```python
from build123d import *

# Parameters (mm, degrees)
SKETCH_W        = 24
SKETCH_H        = 5
PAD_DEPTH       = 5
SKETCH001_R     = 3.75
POCKET_DEPTH    = 2
SKETCH002_R     = 3.75
POCKET001_DEPTH = 2
SKETCH003_R     = 4
POCKET002_DEPTH = 5
SKETCH004_R     = 1.51
POCKET003_DEPTH = 3


with BuildPart() as part:
    # Sketch → Pad (new body)
    with BuildSketch(Plane.XY):
        Rectangle(SKETCH_W, SKETCH_H)
    extrude(amount=PAD_DEPTH)

    # Sketch001 (on Face3 of Pad) → Pocket (cut)
    with BuildSketch(Plane.XZ.offset(2.5)):
        with Locations((0, -2)):
            Circle(SKETCH001_R)
    extrude(amount=-POCKET_DEPTH, mode=Mode.SUBTRACT)

    # Sketch002 (on Face1 of Pocket) → Pocket001 (cut)
    with BuildSketch(Plane(origin=(0, 2.5, 0), x_dir=(-1, 0, 0), z_dir=(0, 1, 0))):
        with Locations((0, -2)):
            Circle(SKETCH002_R)
    extrude(amount=-POCKET001_DEPTH, mode=Mode.SUBTRACT)

    # Sketch003 (on Face7 of Pocket001) → Pocket002 (cut)
    with BuildSketch(Plane.XZ.offset(2.5)):
        with Locations((0, -3)):
            Circle(SKETCH003_R)
        with BuildLine():
            ThreePointArc((4.021194, 2.8), (0, 4.9), (-4.021194, 2.8))
            Line((-4.021194, 2.8), (-12, 2.8))
            Line((-12, 2.8), (-12, 5))
            Line((-12, 5), (12, 5))
            Line((12, 2.8), (12, 5))
            Line((4.021194, 2.8), (12, 2.8))
        make_face()
    extrude(amount=-POCKET002_DEPTH, mode=Mode.SUBTRACT)

    # Sketch004 (on Face8 of Pocket002) → Pocket003 (cut)
    with BuildSketch(Plane.XY.offset(2.8)):
        with Locations((-8, 0)):
            Circle(SKETCH004_R)
        with Locations((8, 0)):
            Circle(SKETCH004_R)
    extrude(amount=-POCKET003_DEPTH, mode=Mode.SUBTRACT)


solid = part.part
```
Source: CAD feature listing. Evaluate the final solid. Frame: model axes, mm. A direction names the side the tool comes from. Coordinates: 2 decimals unless noted, no trailing zeros. Loops run counter-clockwise (first coordinate to the right, second up) from the corner with the lowest first, then second, coordinate; pieces in that order, holes last. Notation, with made-up numbers: M 9,34.5 L 55,34.5 A16 ccw 55,46.5 Z; hole C -33.5,-1 d3. An arc over 180 degrees is marked long. Use a Markdown table: item, result. Add a question column.
Q1. Material intervals for L1, parallel to X at y = -1.05, z = 2.3; L2, parallel to X at y = 1.1, z = 1.45; L3, parallel to Y at x = -8, z = 1.4, sorted ascending.
Q2. Section query C-C, the plane y = -1.85. Return loops of the section in (x, z), and give its area (3 significant figures).
Q3. Section query D-D, the plane z = 2.1. Return loops of the section in (x, y).
Q4. Draft query along X for faces 1 (the cylindrical face through (0.05, -1.51, 1.75)), 2 (the cylindrical face through (0.1, 0, 4.9)), 3 (the flat face through (0, -2.5, 2)). Return one class per face: pulls with the +X half, pulls with the -X half, needs draft (parallel to the pull), parting line crosses it, or undercut.
Q5. Access query for faces 4 (the flat face through (-8, -2, 2.8)), 5 (the cylindrical face through (-0.05, 1.51, 1.75)), 6 (the flat face through (0, -0.5, 1.3)). Directions: +Z, -Z, +X, -X, +Y, -Y. A direction counts if a zero-diameter tool reaches every point of the face in a straight line with its end or side. Return the directions, or none.
Q6. Section query B-B, the plane y = 0. Return loops of the section in (x, z), and give its area (3 significant figures).
Q7. Section query A-A, the plane x = -8. Return loops of the section in (y, z), and give its area (3 significant figures).
Q8. First-contact query: pin 1 (3 mm diameter, centred on x = -2.5, y = -1, fed in from +Z); pin 2 (2.5 mm diameter, centred on x = 8, y = 0, fed in from -Z); pin 3 (1 mm diameter, centred on x = 3.5, y = -1, fed in from +Z); pin 4 (1.9 mm diameter, centred on x = -0.5, z = 0.5, fed in from +Y). Flat tips, straight axial feed; report the tip coordinate or a pass-through.
Result:
| question | item | result |
|---|---|---|
| 1 | L1 | x = -12 to -9.09, -6.91 to 6.91, 9.09 to 12 |
| 1 | L2 | x = -12 to -9.03, -6.97 to -1.47, 1.47 to 6.97, 9.03 to 12 |
| 1 | L3 | y = -2.5 to -1.51, 1.51 to 2.5 |
| 2 | outline | M -12,0 L -3.17,0 A3.75 cw 3.17,0 L 12,0 L 12,2.8 L 4.02,2.8 A4.9 ccw -4.02,2.8 L -12,2.8 Z |
| 2 | area | 71.2 mm2 |
| 3 | outline | M -12,-2.5 L 12,-2.5 L 12,2.5 L -12,2.5 Z; hole C -8,0 d3.02; hole C 8,0 d3.02 |
| 4 | face 1 | undercut |
| 4 | face 2 | parting line crosses it |
| 4 | face 3 | needs draft |
| 5 | face 4 | +Z, -X, +Y, -Y |
| 5 | face 5 | -Z, +Y |
| 5 | face 6 | -Z, -Y |
| 6 | outline | M -12,0 L -9.51,0 L -9.51,2.8 L -12,2.8 Z; M -6.49,0 L -2.65,0 A4 cw 2.65,0 L 6.49,0 L 6.49,2.8 L 4.02,2.8 A4.9 ccw -4.02,2.8 L -6.49,2.8 Z; M 9.51,0 L 12,0 L 12,2.8 L 9.51,2.8 Z |
| 6 | area | 58.5 mm2 |
| 7 | outline | M -2.5,0 L -1.51,0 L -1.51,2.8 L -2.5,2.8 Z; M 1.51,0 L 2.5,0 L 2.5,2.8 L 1.51,2.8 Z |
| 7 | area | 5.54 mm2 |
| 8 | pin 1 | stops at z = 4.8 |
| 8 | pin 2 | passes through |
| 8 | pin 3 | stops at z = 3.87 |
| 8 | pin 4 | stops at y = 0.5 |
